```python
from build123d import *

# Parameters (mm, degrees)
F0_W     = 22.86
F0_H     = 96.774
F1_DEPTH = 18.796
F2_R     = 4.7625
F3_DEPTH = 93.98
F4_R     = 3.175
F5_DEPTH = 12.7


with BuildPart() as f1:
    # F0 (on Top) → F1 (new body)
    with BuildSketch(Plane.XY):
        Rectangle(F0_W, F0_H)
    extrude(amount=F1_DEPTH)

    # F2 (on face) → F3 (cut)
    with BuildSketch(Plane(origin=(0, 48.387, 0), x_dir=(-1, 0, 0), z_dir=(0, 1, 0))):
        with Locations((0, 9.398)):
            Circle(F2_R)
    extrude(amount=-F3_DEPTH, mode=Mode.SUBTRACT)

    # F4 (on face) → F5 (join)
    with BuildSketch(Plane(origin=(0, 0, 0), x_dir=(1, 0, 0), z_dir=(0, 0, -1))):
        with Locations((0, 22.987)):
            Circle(F4_R)
    extrude(amount=F5_DEPTH)


solid = f1.part
```
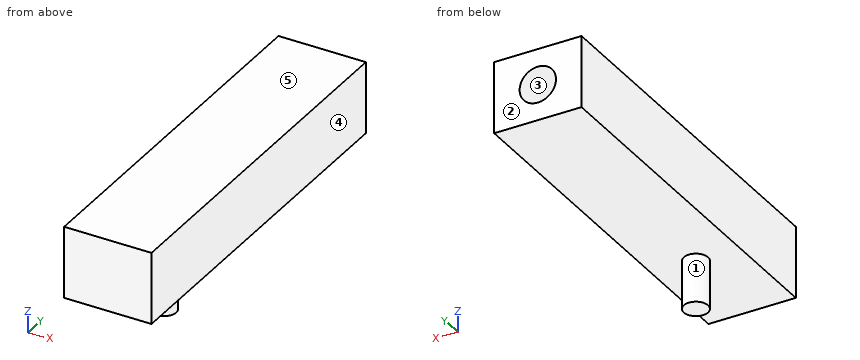
CAD build for the part. Positions are in the model's coordinates, mm. Face numbers are marked on the shaded views. A direction names the side the tool comes from. Round coordinates to 2 decimals unless told otherwise and drop trailing zeros. Write each loop counter-clockwise with the first axis right and the second up, starting at its lowest first coordinate (ties: lowest second). Pieces come first, ordered by that corner, then holes. Notation, with made-up numbers: (39, -13) -> (56, -13) arc R17 cw to (56, 10) -> close; hole circle Ø2 at (-26, -7). An arc over 180 degrees is marked (long way). Answer in a Markdown table with one row per item. Add a question column.
Item 1: Drill centre lines: line 1 (X direction, y = -24, z = 9); line 2 (Z direction, x = 0, y = 10); line 3 (Z direction, x = 0, y = -25). Where is each one in solid material? Low to high. Write a range as from..to.
Item 2: Mould opens along Z. For the marked faces 3, 4 and 5 say: pulls with the +Z half, pulls with the -Z half, needs draft (parallel to the pull), parting line crosses it, or undercut.
Item 3: Saw through at D-D, the plane x = 9.75. Write the cut outline in (y, z).
Item 4: Saw through at B-B, the plane z = 6.5. Write the cut outline in (x, y).
Item 5: Which spindle directions (+Z, -Z, +X, -X, +Y, -Y) get a long thin tool onto all of the face, cutting with end or side? Do the marked faces 1 and 2. Say none if no direction does.
Item 6: Drop flat-ended pins along their axis: pin 1 Ø1.5 at (x, z) = (-1.5, 6.5) entering from +Y; pin 2 Ø7 at (x, y) = (1, -8) entering from -Z. Give the stop position or say it passes through.
Item 7: Saw through at C-C, the plane y = -5.5. Write the cut outline in (x, z) (1 decimal).
Item 8: Saw through at A-A, the plane x = 0. Write the cut outline in (y, z), then the cut area to 3 significant figures.
Findings below:
| question | item | result |
|---|---|---|
| 1 | line 1 | x = -11.43..-4.75, 4.75..11.43 |
| 1 | line 2 | z = 0..4.64, 14.16..18.8 |
| 1 | line 3 | z = -12.7..4.64, 14.16..18.8 |
| 2 | face 3 | undercut |
| 2 | face 4 | needs draft |
| 2 | face 5 | pulls with the +Z half |
| 3 | outline | (-48.39, 0) -> (48.39, 0) -> (48.39, 18.8) -> (-48.39, 18.8) -> close |
| 4 | outline | (-11.43, -48.39) -> (11.43, -48.39) -> (11.43, 48.39) -> (3.78, 48.39) -> (3.78, -45.59) -> (-3.78, -45.59) -> (-3.78, 48.39) -> (-11.43, 48.39) -> close |
| 5 | face 1 | -Z |
| 5 | face 2 | +Z, -Z, +X, -X, +Y |
| 6 | pin 1 | stops at y = -45.59 |
| 6 | pin 2 | stops at z = 0 |
| 7 | outline | (-11.4, 0) -> (11.4, 0) -> (11.4, 18.8) -> (-11.4, 18.8) -> close; hole circle Ø9.5 at (0, 9.4) |
| 8 | outline | (-48.39, 0) -> (-26.16, 0) -> (-26.16, -12.7) -> (-19.81, -12.7) -> (-19.81, 0) -> (48.39, 0) -> (48.39, 4.64) -> (-45.59, 4.64) -> (-45.59, 14.16) -> (48.39, 14.16) -> (48.39, 18.8) -> (-48.39, 18.8) -> close |
| 8 | area | 1,000 mm^2 |
